from build123d import *

# Parameters (mm, degrees)
SKETCH1_W               = 498
SKETCH1_H               = 37
BOSS_EXTRUDE1_DEPTH     = 27
SKETCH3_W               = 30
SKETCH3_H               = 27
CUT_EXTRUDE2_DEPTH      = 4
SKETCH4_W               = 77.8
SKETCH4_H               = 23
CUT_EXTRUDE3_DEPTH      = 28
SKETCH5_W               = 77.8
SKETCH5_H               = 7.65
CUT_EXTRUDE4_DEPTH      = 15
SKETCH6_W               = 16
SKETCH6_H               = 14
CUT_EXTRUDE5_DEPTH      = 3.05
CUT_EXTRUDE6_DEPTH      = 1
M3_TAPPED_HOLE1_D       = 2.5
M3_TAPPED_HOLE1_DEPTH   = 6
M3_TAPPED_HOLE1_TIP     = 0.751075774
M4_TAPPED_HOLE1_D       = 3.3
M4_TAPPED_HOLE1_DEPTH   = 8
M4_TAPPED_HOLE1_TIP     = 0.991420021
M3_TAPPED_HOLE2_D       = 2.5
M3_TAPPED_HOLE2_DEPTH   = 6
M3_TAPPED_HOLE2_TIP     = 0.751075774
M3_TAPPED_HOLE3_D       = 2.5
M3_TAPPED_HOLE3_DEPTH   = 6
M3_TAPPED_HOLE3_TIP     = 0.751075774
SKETCH16_W              = 10
SKETCH16_H              = 33
CUT_EXTRUDE7_DEPTH      = 0.4
FILLET1_R               = 1
CHAMFER1_SIZE           = 0.5
FILLET2_R               = 1
CHAMFER2_SIZE           = 5
SKETCH17_R              = 1.5
CUT_EXTRUDE8_DEPTH      = 6
SKETCH19_R              = 6.347203473
SKETCH19_R_2            = 6.528534634
CUT_EXTRUDE9_DEPTH      = 28
M3_5_TAPPED_HOLE1_D     = 2.9
M3_5_TAPPED_HOLE1_DEPTH = 5
M3_5_TAPPED_HOLE1_TIP   = 0.871247898
M4_TAPPED_HOLE3_D       = 3.3
M4_TAPPED_HOLE3_DEPTH   = 7
M4_TAPPED_HOLE3_TIP     = 0.991420021


with BuildPart() as part:
    # Sketch1 → Boss-Extrude1 (new body)
    with BuildSketch(Plane.XY):
        with Locations((97.902272727, 23.094318182)):
            Rectangle(SKETCH1_W, SKETCH1_H)
    extrude(amount=BOSS_EXTRUDE1_DEPTH)

    # Sketch3 → Cut-Extrude2 (cut)
    with BuildSketch(Plane(origin=(0, 0, 0), x_dir=(-1, 0, 0), z_dir=(0, 0, -1))):
        with Locations((-279.902272727, 18.094318182)):
            Rectangle(SKETCH3_W, SKETCH3_H)
    extrude(amount=-CUT_EXTRUDE2_DEPTH, mode=Mode.SUBTRACT)

    # Sketch4 → Cut-Extrude3 (cut, through all)
    with BuildSketch(Plane(origin=(0, 0, 0), x_dir=(-1, 0, 0), z_dir=(0, 0, -1))):
        with Locations((-24.902272727, 30.094318182)):
            Rectangle(SKETCH4_W, SKETCH4_H)
    extrude(amount=-CUT_EXTRUDE3_DEPTH, mode=Mode.SUBTRACT)

    # Sketch5 → Cut-Extrude4 (cut, through all)
    with BuildSketch(Plane(origin=(0, 18.594318182, 0), x_dir=(1, 0, 0), z_dir=(0, 1, 0))):
        with Locations((24.902272727, -3.825)):
            Rectangle(SKETCH5_W, SKETCH5_H)
    extrude(amount=-CUT_EXTRUDE4_DEPTH, mode=Mode.SUBTRACT)

    # Sketch6 → Cut-Extrude5 (cut)
    with BuildSketch(Plane(origin=(0, 0, 7.65), x_dir=(-1, 0, 0), z_dir=(0, 0, -1))):
        with Locations((-24.902272727, 11.594318182)):
            Rectangle(SKETCH6_W, SKETCH6_H)
    extrude(amount=-CUT_EXTRUDE5_DEPTH, mode=Mode.SUBTRACT)

    # Sketch7 → Cut-Extrude6 (cut)
    with BuildSketch(Plane(origin=(0, 0, 0), x_dir=(-1, 0, 0), z_dir=(0, 0, -1))):
        Polygon((151.097727273, 36.25457222), (146.097727273, 37.594318182), (18.242292409, 37.594318182), (13.997727273, 36.456990381), (13.997727273, 37.594318182), (-63.802272727, 37.594318182), (-341.902272727, 37.594318182), (-346.902272727, 36.25457222), (-346.902272727, 41.594318182), (151.097727273, 41.594318182), align=None)
    extrude(amount=-CUT_EXTRUDE6_DEPTH, mode=Mode.SUBTRACT)

    # M3 Tapped Hole1
    with Locations(Plane(origin=(0, 4.594318182, 0), x_dir=(-1, 0, 0), z_dir=(0, -1, 0))):
        with Locations((-286.402272727, -11.76), (-273.402272727, -11.76)):
            Hole(M3_TAPPED_HOLE1_D / 2, depth=M3_TAPPED_HOLE1_DEPTH)
            with Locations((0, 0, -(M3_TAPPED_HOLE1_DEPTH + M3_TAPPED_HOLE1_TIP / 2))):  # 118° drill point
                Cone(0, M3_TAPPED_HOLE1_D / 2, M3_TAPPED_HOLE1_TIP, mode=Mode.SUBTRACT)

    # M4 Tapped Hole1
    with Locations(Plane(origin=(0, 0, 7.65), x_dir=(-1, 0, 0), z_dir=(0, 0, -1))):
        with Locations((5.097727273, 11.594318182), (-54.902272727, 11.594318182)):
            Hole(M4_TAPPED_HOLE1_D / 2, depth=M4_TAPPED_HOLE1_DEPTH)
            with Locations((0, 0, -(M4_TAPPED_HOLE1_DEPTH + M4_TAPPED_HOLE1_TIP / 2))):  # 118° drill point
                Cone(0, M4_TAPPED_HOLE1_D / 2, M4_TAPPED_HOLE1_TIP, mode=Mode.SUBTRACT)

    # M3 Tapped Hole2
    with Locations(Plane(origin=(0, 0, 0), x_dir=(-1, 0, 0), z_dir=(0, 0, -1))):
        with Locations((71.097727273, 31.594318182), (41.097727273, 31.594318182), (-99.902272727, 31.594318182), (-151.902272727, 31.594318182), (-206.902272727, 31.594318182), (-221.902272727, 31.594318182), (-354.592417471, -112.457729383)):
            Hole(M3_TAPPED_HOLE2_D / 2, depth=M3_TAPPED_HOLE2_DEPTH)
            with Locations((0, 0, -(M3_TAPPED_HOLE2_DEPTH + M3_TAPPED_HOLE2_TIP / 2))):  # 118° drill point
                Cone(0, M3_TAPPED_HOLE2_D / 2, M3_TAPPED_HOLE2_TIP, mode=Mode.SUBTRACT)

    # M3 Tapped Hole3
    with Locations(Plane(origin=(0, 4.594318182, 0), x_dir=(-1, 0, 0), z_dir=(0, -1, 0))):
        with Locations((12.397727273, -14.1), (4.397727273, -14.1)):
            Hole(M3_TAPPED_HOLE3_D / 2, depth=M3_TAPPED_HOLE3_DEPTH)
            with Locations((0, 0, -(M3_TAPPED_HOLE3_DEPTH + M3_TAPPED_HOLE3_TIP / 2))):  # 118° drill point
                Cone(0, M3_TAPPED_HOLE3_D / 2, M3_TAPPED_HOLE3_TIP, mode=Mode.SUBTRACT)

    # Sketch16 → Cut-Extrude7 (cut)
    with BuildSketch(Plane(origin=(0, 0, 0), x_dir=(-1, 0, 0), z_dir=(0, 0, -1))):
        with Locations((-84.402272727, 21.094318182)):
            Rectangle(SKETCH16_W, SKETCH16_H)
    extrude(amount=-CUT_EXTRUDE7_DEPTH, mode=Mode.SUBTRACT)

    # Fillet1
    fillet1_edges = [part.edges().sort_by_distance(p)[0] for p in [
        (-13.997727273, 18.594318182, 17.325),
        (63.802272727, 18.594318182, 17.325),
    ]]
    fillet(fillet1_edges, radius=FILLET1_R)

    # Chamfer1
    chamfer1_edges = [part.edges().sort_by_distance(p)[0] for p in [
        (16.902272727, 11.594318182, 7.65),
        (32.902272727, 11.594318182, 7.65),
    ]]
    chamfer(chamfer1_edges, length=CHAMFER1_SIZE)

    # Fillet2
    fillet2_edges = [part.edges().sort_by_distance(p)[0] for p in [
        (264.902272727, 31.594318182, 2),
        (294.902272727, 31.594318182, 2),
    ]]
    fillet(fillet2_edges, radius=FILLET2_R)

    # Chamfer2
    chamfer2_edges = [part.edges().sort_by_distance(p)[0] for p in [
        (346.902272727, 4.594318182, 13.5),
        (-151.097727273, 4.594318182, 13.5),
    ]]
    chamfer(chamfer2_edges, length=CHAMFER2_SIZE)

    # Sketch17 → Cut-Extrude8 (cut)
    with BuildSketch(Plane(origin=(0, 0, 0), x_dir=(-1, 0, 0), z_dir=(0, 0, -1))):
        with Locations((-323.902272727, 27.594318182)):
            Circle(SKETCH17_R)
        with Locations((-337.902272727, 27.594318182)):
            Circle(SKETCH17_R)
    extrude(amount=-CUT_EXTRUDE8_DEPTH, mode=Mode.SUBTRACT)

    # Sketch19 → Cut-Extrude9 (cut, through all)
    with BuildSketch(Plane.XY.offset(27)):
        with Locations((-139.197727273, 21.594318182)):
            Circle(SKETCH19_R)
        with Locations((-22.197727273, 21.594318182)):
            Circle(SKETCH19_R_2)
        with Locations((150.802272727, 21.594318182)):
            Circle(SKETCH19_R)
        with Locations((323.802272727, 21.594318182)):
            Circle(SKETCH19_R)
    extrude(amount=-CUT_EXTRUDE9_DEPTH, mode=Mode.SUBTRACT)

    # M3.5 Tapped Hole1
    with Locations(Plane(origin=(0, 4.594318182, 0), x_dir=(-1, 0, 0), z_dir=(0, -1, 0))):
        with Locations((-131.42052192, -2.174485534), (-131.42052192, -14.174485534), (-81.42052192, -2.174485534)):
            Hole(M3_5_TAPPED_HOLE1_D / 2, depth=M3_5_TAPPED_HOLE1_DEPTH)
            with Locations((0, 0, -(M3_5_TAPPED_HOLE1_DEPTH + M3_5_TAPPED_HOLE1_TIP / 2))):  # 118° drill point
                Cone(0, M3_5_TAPPED_HOLE1_D / 2, M3_5_TAPPED_HOLE1_TIP, mode=Mode.SUBTRACT)

    # M4 Tapped Hole3
    with Locations(Plane(origin=(0, 0, 0), x_dir=(-1, 0, 0), z_dir=(0, 0, -1))):
        with Locations((-246.689139378, 8.594318182), (-246.689139378, 20.594318182)):
            Hole(M4_TAPPED_HOLE3_D / 2, depth=M4_TAPPED_HOLE3_DEPTH)
            with Locations((0, 0, -(M4_TAPPED_HOLE3_DEPTH + M4_TAPPED_HOLE3_TIP / 2))):  # 118° drill point
                Cone(0, M4_TAPPED_HOLE3_D / 2, M4_TAPPED_HOLE3_TIP, mode=Mode.SUBTRACT)


solid = part.part
Here's how the part is built. I have some questions about the finished solid (model axes, mm). A direction names the side the tool comes from. Coordinates: 2 decimals unless noted, no trailing zeros.
1) Which directions (+Z, -Z, +X, -X, +Y, -Y) give clear straight access to the entire face, cutting with the end or side of a thin tool? Please do faces 1 (the face through (280, 18, 4)), 2 (the face through (63.802, 27, 11)), 3 (the face through (25, 12, 10.7)), 4 (the face through (94, 23, 27)), 5 (the face through (25, 18.594, 17)).
Filled in:
face 1: -Z, -Y
face 2: -Z, +Y
face 3: -Z, +Y, -Y
face 4: +Z, +X, -X, +Y, -Y
face 5: +Z, -Z, +Y
2) I'm going to push flat-ended pins straight in: pin 1 (7.5 mm diameter, centred on x = 55.5, y = 15.5, fed in from -Z); pin 2 (2 mm diameter, centred on x = -41.1, y = 31.59, fed in from -Z); pin 3 (6 mm diameter, centred on x = 17, z = 13, fed in from +Y). Where does each tip first touch, or does it pass through?
Filled in:
pin 1: stops at z = 7.65
pin 2: stops at z = 6.15
pin 3: stops at y = 18.59
3) If I drill on line 1 (X direction, y = 21.5, z = 12.5); line 2 (X direction, y = 24, z = 23.5); line 3 (X direction, y = 9.5, z = 9.75), over which ranges is the centre line in solid material (lowest first)?
Filled in:
line 1: x = -151.1 to -145.54, -132.85 to -28.73, -15.67 to -14, 63.8 to 144.46, 157.15 to 317.46, 330.15 to 346.9
line 2: x = -151.1 to -145.07, -133.32 to -28.27, -16.13 to -14, 63.8 to 144.93, 156.68 to 317.93, 329.68 to 346.9
line 3: x = -151 to 16.9, 32.9 to 346.81
4) Thinking about a two-plate mould opening in Y: for faces 6 (the face through (144.46, 21.87, 13.69)), 7 (the face through (203, 41.594, 14)), 8 (the face through (-84, 21, 0)), which applies, +Y half, -Y half, draft (parallel to the pull), parting line (faces both ways), or undercut?
Filled in:
face 6: undercut
face 7: +Y half
face 8: draft
